from build123d import *

# Parameters (mm, degrees)
SKETCH1_W           = 40
SKETCH1_H           = 40
SKETCH1_W_2         = 35
SKETCH1_H_2         = 35
BOSS_EXTRUDE1_DEPTH = 30
SKETCH2_W           = 40
SKETCH2_H           = 40
BOSS_EXTRUDE2_DEPTH = 2.5
SKETCH3_W           = 35
SKETCH3_H           = 20
CUT_EXTRUDE1_DEPTH  = 2.5
FILLET1_R           = 1
FILLET2_R           = 1
BOSS_EXTRUDE3_DEPTH = 2.5
BOSS_EXTRUDE4_DEPTH = 2.5


with BuildPart() as part:
    # Sketch1 → Boss-Extrude1 (new body)
    with BuildSketch(Plane(origin=(0, 0, 0), x_dir=(1, 0, 0), z_dir=(0, 1, 0))):
        Rectangle(SKETCH1_W, SKETCH1_H)
        Rectangle(SKETCH1_W_2, SKETCH1_H_2, mode=Mode.SUBTRACT)
    extrude(amount=BOSS_EXTRUDE1_DEPTH)

    # Sketch2 → Boss-Extrude2 (add)
    with BuildSketch(Plane(origin=(0, 0, 0), x_dir=(1, 0, 0), z_dir=(0, 1, 0))):
        Rectangle(SKETCH2_W, SKETCH2_H)
    extrude(amount=BOSS_EXTRUDE2_DEPTH)

    # Sketch3 → Cut-Extrude1 (cut)
    with BuildSketch(Plane(origin=(20, 0, 0), x_dir=(0, 0, -1), z_dir=(1, 0, 0))):
        with Locations((0, 20)):
            Rectangle(SKETCH3_W, SKETCH3_H)
    extrude(amount=-CUT_EXTRUDE1_DEPTH, mode=Mode.SUBTRACT)

    # Fillet1
    fillet1_edges = [part.edges().sort_by_distance(p)[0] for p in [
        (20, 15, 20),
        (-20, 15, 20),
    ]]
    fillet(fillet1_edges, radius=FILLET1_R)

    # Fillet2
    fillet2_edges = [part.edges().sort_by_distance(p)[0] for p in [
        (-20, 15, -20),
        (20, 15, -20),
    ]]
    fillet(fillet2_edges, radius=FILLET2_R)

    # Sketch4 → Boss-Extrude3 (add)
    with BuildSketch(Plane.XY.offset(20)):
        with BuildLine():
            ThreePointArc((-3.5, 30), (-2.474873734, 32.474873734), (0, 33.5))
            Line((0, 33.5), (0, 35))
            ThreePointArc((0, 35), (-3.535533906, 33.535533906), (-5, 30))
            Line((-5, 30), (-3.5, 30))
        make_face()
        with BuildLine():
            Line((0, 35), (0, 33.5))
            ThreePointArc((0, 33.5), (2.474873734, 32.474873734), (3.5, 30))
            Line((3.5, 30), (5, 30))
            ThreePointArc((5, 30), (3.535533906, 33.535533906), (0, 35))
        make_face()
    extrude(amount=-BOSS_EXTRUDE3_DEPTH)

    # Sketch5 → Boss-Extrude4 (add)
    with BuildSketch(Plane(origin=(0, 0, -20), x_dir=(-1, 0, 0), z_dir=(0, 0, -1))):
        with BuildLine():
            ThreePointArc((-3.5, 30), (-2.474873734, 32.474873734), (0, 33.5))
            Line((0, 33.5), (0, 35))
            ThreePointArc((0, 35), (-3.535533906, 33.535533906), (-5, 30))
            Line((-5, 30), (-3.5, 30))
        make_face()
        with BuildLine():
            Line((0, 35), (0, 33.5))
            ThreePointArc((0, 33.5), (2.474873734, 32.474873734), (3.5, 30))
            Line((3.5, 30), (5, 30))
            ThreePointArc((5, 30), (3.535533906, 33.535533906), (0, 35))
        make_face()
    extrude(amount=-BOSS_EXTRUDE4_DEPTH)


solid = part.part
Can you work these out from the model? Positions are in its coordinate system, mm. A direction names the side the tool comes from. Coordinates: 2 decimals unless noted, no trailing zeros. Write each loop counter-clockwise with the first axis right and the second up, starting at its lowest first coordinate (ties: lowest second). Pieces come first, ordered by that corner, then holes. Notation, with made-up numbers: (-22, -1.75) - (24, -1.75) arc R25 ccw to (24, 17.25) - close; hole circle Ø6 at (-30.75, 4). An arc over 180 degrees is marked (long way). Return JSON: item names as keys, results as strings. Group by question number.
Item 1: If we section it at A-A (z = -9): Write out the boundary of the cut face in (x, y).
Item 2: I'm going to push flat-ended pins straight in: pin 1 Ø16.5 at (x, z) = (-13.5, 5) entering from +Y; pin 2 Ø2 at (y, z) = (24, -5) entering from +X; pin 3 Ø1.2 at (x, z) = (19, 7.5) entering from +Y. Where does each tip first touch, or does it pass through?
Item 3: Please list where these lines run through material, in increasing order: probe 1 along Z at (x, y) = (-3, 19.5); probe 2 along Y at (x, z) = (9, 2.5).
Item 4: If we section it at D-D (y = 32): Write out the boundary of the cut face in (x, z).
Item 5: We'd pull the mould along Z, two halves only. Please class faces 4 (the face through (-17.5, 16, 0)), 5 (the face through (0, 0, 0)), 6 (the face through (-19.715, 14.79, -19.699)): pulls with the +Z half, pulls with the -Z half, needs draft (parallel to the pull), parting line crosses it, or undercut.
Item 6: If we section it at B-B (x = 2): Write out the boundary of the cut face in (y, z), then the cut area to 3 significant figures.
Item 7: Which directions (+Z, -Z, +X, -X, +Y, -Y) give clear straight access to the entire face, cutting with the end or side of a thin tool? Please do faces 1 (the face through (12, 30, -19)), 2 (the face through (2, 19, -17.5)), 3 (the face through (0, 30, -19)).
Item 8: If we section it at C-C (y = 23): Write out the boundary of the cut face in (x, z), then the cut area to 3 significant figures.
Return value:
{
 "1": {"outline": "(-20, 0) - (20, 0) - (20, 10) - (17.5, 10) - (17.5, 2.5) - (-17.5, 2.5) - (-17.5, 30) - (-20, 30) - close"},
 "2": {"pin 1": "stops at y = 30", "pin 2": "stops at x = -17.5", "pin 3": "stops at y = 10"},
 "3": {"probe 1": "z = -20 to -17.5, 17.5 to 20", "probe 2": "y = 0 to 2.5"},
 "4": {"outline": "(-4.58, -20) - (-2.87, -20) - (-2.87, -17.5) - (-4.58, -17.5) - close; (-4.58, 17.5) - (-2.87, 17.5) - (-2.87, 20) - (-4.58, 20) - close; (2.87, -20) - (4.58, -20) - (4.58, -17.5) - (2.87, -17.5) - close; (2.87, 17.5) - (4.58, 17.5) - (4.58, 20) - (2.87, 20) - close"},
 "5": {"face 4": "undercut", "face 5": "needs draft", "face 6": "pulls with the -Z half"},
 "6": {"outline": "(0, -20) - (30, -20) - (30, -17.5) - (2.5, -17.5) - (2.5, 17.5) - (30, 17.5) - (30, 20) - (0, 20) - close; (32.87, -20) - (34.58, -20) - (34.58, -17.5) - (32.87, -17.5) - close; (32.87, 17.5) - (34.58, 17.5) - (34.58, 20) - (32.87, 20) - close", "area": "246 mm^2"},
 "7": {"face 1": "+Z, -Z, +X, +Y", "face 2": "+Y", "face 3": "+Z, -Z"},
 "8": {"outline": "(-20, -19) arc R1 ccw to (-19, -20) - (19, -20) arc R1 ccw to (20, -19) - (20, -17.5) - (-17.5, -17.5) - (-17.5, 17.5) - (20, 17.5) - (20, 19) arc R1 ccw to (19, 20) - (-19, 20) arc R1 ccw to (-20, 19) - close", "area": "287 mm^2"}
}
